```python
from build123d import *

# Parameters (mm, degrees)
F2_R     = 10.16
F2_R_2   = 6.35
F3_DEPTH = 1.27


with BuildPart() as f1:
    # F0 (on Front) → F1 (revolve)
    with BuildSketch(Plane.XZ):
        with BuildLine():
            Line((0, 2.54), (0, 0))
            Line((0, 0), (10.16, 0))
            Line((10.16, 0), (10.16, 2.54))
            Line((10.16, 2.54), (4, 2.54))
            Line((4, 2.54), (4, 9.54))
            Line((4, 9.54), (2.75, 9.54))
            Line((2.75, 9.54), (2.75, 5.564))
            ThreePointArc((2.75, 5.564), (3.181095, 4.802), (2.75, 4.04))
            Line((2.75, 4.04), (2.75, 2.54))
            Line((2.75, 2.54), (0, 2.54))
        make_face()
    revolve(axis=Axis((0, 0, 1.27), (0, 0, -1)))

    # F2 (on face) → F3 (cut)
    with BuildSketch(Plane.XY.offset(2.54)):
        Circle(F2_R)
        Circle(F2_R_2, mode=Mode.SUBTRACT)
    extrude(amount=-F3_DEPTH, mode=Mode.SUBTRACT)


solid = f1.part
```
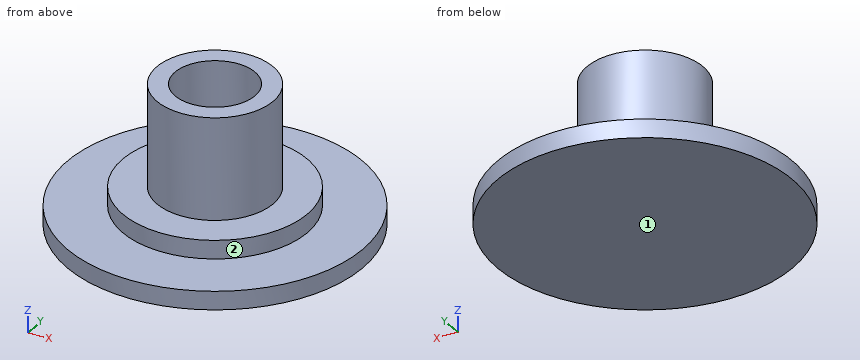
Geometry: final body of the model. Coordinates: model frame, mm. Face numbers are marked on the shaded views. A direction names the side the tool comes from. Round coordinates to 2 decimals unless told otherwise and drop trailing zeros. Order: outer loops, then holes, each group sorted by start corner. A loop starts at its lowest first (then second) coordinate and runs counter-clockwise, first axis right, second up. Notation, with made-up numbers: (-29.5, 42) - (29.5, 42) arc R19 ccw to (29.5, 49) - close; hole circle Ø8 at (87.25, 11.5). An arc over 180 degrees is marked (long way). Use CSV: the item, a comma, the result in double quotes. Start each with the question number.
Q1. Access query for the marked faces 1 and 2. Directions: +Z, -Z, +X, -X, +Y, -Y. A direction counts if a zero-diameter tool reaches every point of the face in a straight line with its end or side. Return the directions, or none.
Q2. Section query D-D (y = 7.75). Return loops of the section in (x, z), and give its area (3 significant figures).
Q3. Section query C-C (z = 2). Return loops of the section in (x, y).
Q4. First-contact query: pin 1 (5 mm diameter, centred on x = -4.5, z = 5.5, fed in from -Y); pin 2 (5 mm diameter, centred on y = -6, z = 8, fed in from +X). Flat tips, straight axial feed; report the tip coordinate or a pass-through.
Q5. Section query A-A (x = 0). Return loops of the section in (y, z).
Q6. Section query B-B (z = 6). Return loops of the section in (x, y), and give its area (3 significant figures).
Q7. Material intervals for line 1 along Y through (x, z) = (0, 7); line 2 along Z through (x, y) = (-5.5, -8.5), sorted ascending. Write a range as from..to.
Result set:
1,face 1,"-Z, +X, -X, +Y, -Y"
1,face 2,"+Z"
2,outline,"(-6.57, 0) - (6.57, 0) - (6.57, 1.27) - (-6.57, 1.27) - close"
2,area,"16.7 mm2"
3,outline,"circle Ø12.7 at (0, 0)"
4,pin 1,"stops at y = -3.46"
4,pin 2,"stops at x = 1.94"
5,outline,"(-10.16, 0) - (10.16, 0) - (10.16, 1.27) - (6.35, 1.27) - (6.35, 2.54) - (4, 2.54) - (4, 9.54) - (2.75, 9.54) - (2.75, 5.56) arc R0.89 cw to (2.75, 4.04) - (2.75, 2.54) - (-2.75, 2.54) - (-2.75, 4.04) arc R0.89 cw to (-2.75, 5.56) - (-2.75, 9.54) - (-4, 9.54) - (-4, 2.54) - (-6.35, 2.54) - (-6.35, 1.27) - (-10.16, 1.27) - close"
6,outline,"circle Ø8 at (0, 0); hole circle Ø5.5 at (0, 0)"
6,area,"26.5 mm2"
7,line 1,"y = -4..-2.75, 2.75..4"
7,line 2,"z = 0..1.27"
